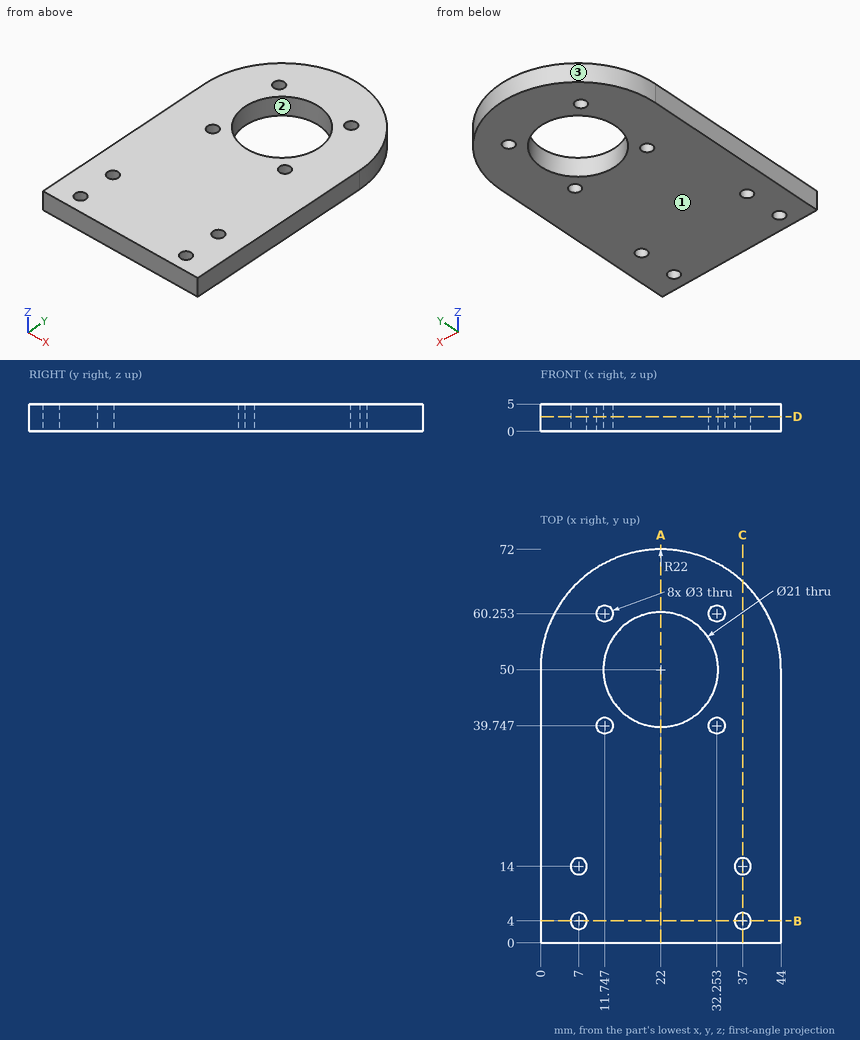
Geometry check sheet. Reference: drawing and pictorial views, mm from the part's lowest x, y, z. Give positions to 0.01 mm unless a question says otherwise; leave off trailing zeros. Order: outer loops, then holes, each group sorted by start corner. A loop starts at its lowest first (then second) coordinate and runs counter-clockwise, first axis right, second up.
1. Section check A-A, the plane x = 22. Enter the section's corners in (y, z), and give its area (3 significant figures).
2. Gauge pin test, flat ends, axial feed: pin 1 Ø1.8 at (x, y) = (11.75, 39.75) entering from -Z (3 decimals); pin 2 Ø2 at (x, z) = (14, 1) entering from +Y; pin 3 Ø1 at (x, z) = (24.5, 2.5) entering from +Y. Record the tip position at first contact, or that the pin passes through.
3. Section check D-D, the plane z = 2.7. Give the number of separate pieces and of enclosed holes in the cut face, and give its area (3 significant figures).
4. Section check C-C, the plane x = 37. Enter the section's corners in (y, z).
5. Release check for a two-part mould opening along X. For the marked faces 1, 2 and 3 record: pulls with the +X half, pulls with the -X half, needs draft (parallel to the pull), parting line crosses it, or undercut.
6. Thickness scan on L1, parallel to Y at x = 33.5, z = 0.4 (1 decimal); L2, parallel to Y at x = 22, z = 3.5; L3, parallel to Y at x = 37.5, z = 1.75. Record the ranges inside material, lowest first.
7. Section check B-B, the plane y = 4. Enter the section's corners in (x, z), and give its area (3 significant figures).
Values follow:
1. outline: (0, 0) - (39.5, 0) - (39.5, 5) - (0, 5) - close; (60.5, 0) - (72, 0) - (72, 5) - (60.5, 5) - close
1. area: 255 mm2
2. pin 1: passes through
2. pin 2: stops at y = 70.86
2. pin 3: stops at y = 71.91
3. separate pieces: 1
3. enclosed holes: 9
3. area: 2,560 mm2
4. outline: (0, 0) - (2.5, 0) - (2.5, 5) - (0, 5) - close; (5.5, 0) - (12.5, 0) - (12.5, 5) - (5.5, 5) - close; (15.5, 0) - (66.09, 0) - (66.09, 5) - (15.5, 5) - close
5. face 1: needs draft
5. face 2: undercut
5. face 3: parting line crosses it
6. L1: y = 0 to 38.9, 40.6 to 59.4, 61.1 to 68.8
6. L2: y = 0 to 39.5, 60.5 to 72
6. L3: y = 0 to 2.59, 5.41 to 12.59, 15.41 to 65.61
7. outline: (0, 0) - (5.5, 0) - (5.5, 5) - (0, 5) - close; (8.5, 0) - (35.5, 0) - (35.5, 5) - (8.5, 5) - close; (38.5, 0) - (44, 0) - (44, 5) - (38.5, 5) - close
7. area: 190 mm2
